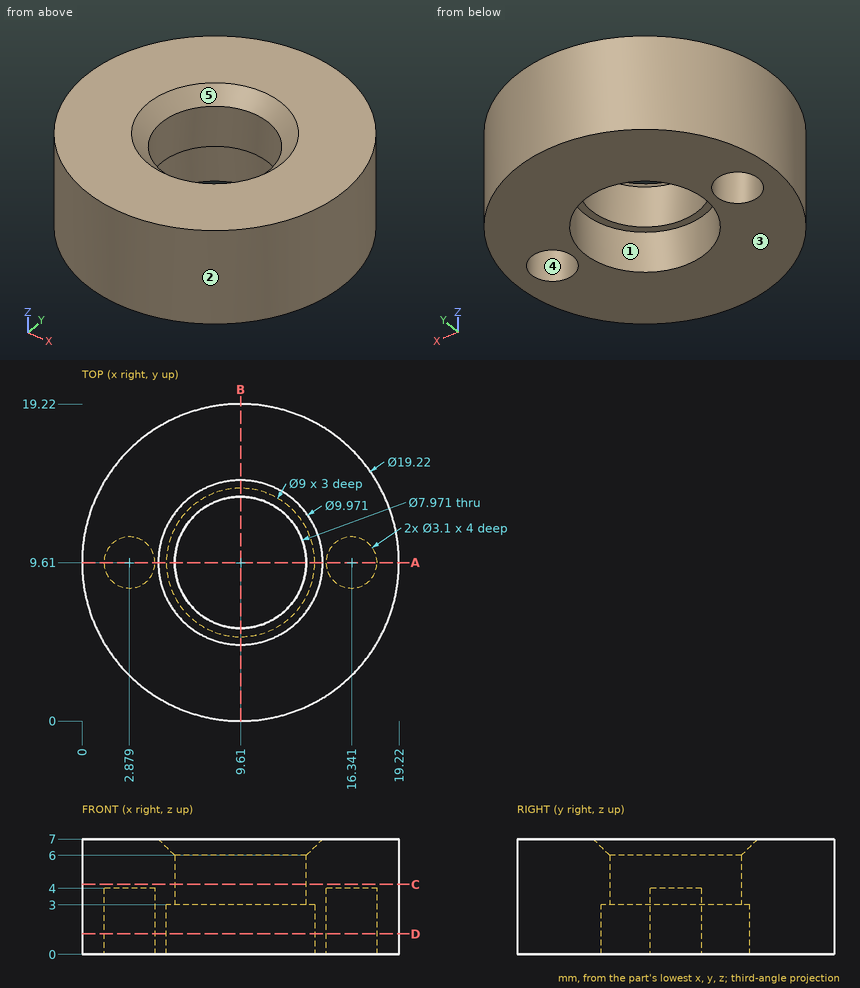
Can you work these out from the drawing? Everything is in mm from the part's minimum corner. A direction names the side the tool comes from. Give positions to 0.01 mm unless a question says otherwise; leave off trailing zeros. Write each loop counter-clockwise with the first axis right and the second up, starting at its lowest first coordinate (ties: lowest second). Pieces come first, ordered by that corner, then holes. Notation, with made-up numbers: M 29.25,30.25 L 45.25,30.25 A16 cw 45.25,45.25 Z; hole C -17,3.25 d6. An arc over 180 degrees is marked long. Answer in a Markdown table with one row per item. Add a question column.
Item 1: Imagine slicing it at D-D, the plane z = 1.25. Write out the boundary of the cut face in (x, y).
Item 2: Imagine slicing it at A-A, the plane y = 9.61. Write out the boundary of the cut face in (x, z) (1 decimal).
Item 3: Imagine slicing it at C-C, the plane z = 4.25. Write out the boundary of the cut face in (x, y) (1 decimal).
Item 4: On a 3-axis mill with a long thin cutter (end or side, diameter ignored), from which of +Z, -Z, +X, -X, +Y, -Y can I reach the whole of each face in a straight line? I mean the marked faces 4 and 5. Say none if no direction works.
Item 5: Please list where these lines run through material, in increasing order: L1, parallel to X at y = 9.5, z = 5 (1 decimal); L2, parallel to Y at x = 9.61, z = 0.7.
Item 6: Imagine slicing it at B-B, the plane x = 9.61. Write out the boundary of the cut face in (y, z) (1 decimal).
Item 7: We'd pull the mould along X, two halves only. Please class the marked faces 1, 2 and 3: released by +X, released by -X, zero draft, split by the parting line, or undercut.
Item 8: For pin 1 Ø3 at (x, y) = (2.88, 9.61) entering from -Z; pin 2 Ø4 at (x, y) = (12, 3.5) entering from -Z; pin 3 Ø2 at (x, z) = (7.5, 1.5) entering from +Y; pin 4 Ø1 at (x, z) = (12.5, 1.5) entering from +Y, each with a flat end and sliding along its axis, tell me the tip position at first contact or that it passes through.
Evaluation:
| question | item | result |
|---|---|---|
| 1 | outline | C 9.61,9.61 d19.22; hole C 2.88,9.61 d3.1; hole C 9.61,9.61 d9; hole C 16.34,9.61 d3.1 |
| 2 | outline | M 0,0 L 1.3,0 L 1.3,4 L 4.4,4 L 4.4,0 L 5.1,0 L 5.1,3 L 5.6,3 L 5.6,6 L 4.6,7 L 0,7 Z; M 13.6,3 L 14.1,3 L 14.1,0 L 14.8,0 L 14.8,4 L 17.9,4 L 17.9,0 L 19.2,0 L 19.2,7 L 14.6,7 L 13.6,6 Z |
| 3 | outline | C 9.6,9.6 d19.2; hole C 9.6,9.6 d8 |
| 4 | face 4 | -Z |
| 4 | face 5 | +Z |
| 5 | L1 | x = 0 to 5.6, 13.6 to 19.2 |
| 5 | L2 | y = 0 to 5.11, 14.11 to 19.22 |
| 6 | outline | M 0,0 L 5.1,0 L 5.1,3 L 5.6,3 L 5.6,6 L 4.6,7 L 0,7 Z; M 13.6,3 L 14.1,3 L 14.1,0 L 19.2,0 L 19.2,7 L 14.6,7 L 13.6,6 Z |
| 7 | face 1 | undercut |
| 7 | face 2 | split by the parting line |
| 7 | face 3 | zero draft |
| 8 | pin 1 | stops at z = 4 |
| 8 | pin 2 | stops at z = 0 |
| 8 | pin 3 | stops at y = 19.16 |
| 8 | pin 4 | stops at y = 18.92 |
